Geometry: see drawing. Coordinates: mm, zero at the bounding-box minimum. Coordinates: 2 decimals unless noted, no trailing zeros. Write each loop counter-clockwise with the first axis right and the second up, starting at its lowest first coordinate (ties: lowest second). Pieces come first, ordered by that corner, then holes. Notation, with made-up numbers: (12, 86.25) - (62, 86.25) arc R9 cw to (62, 101.25) - close; hole circle Ø4 at (-12, 83). An arc over 180 degrees is marked (long way). Use CSV: the item, a comma, the result in double quotes.
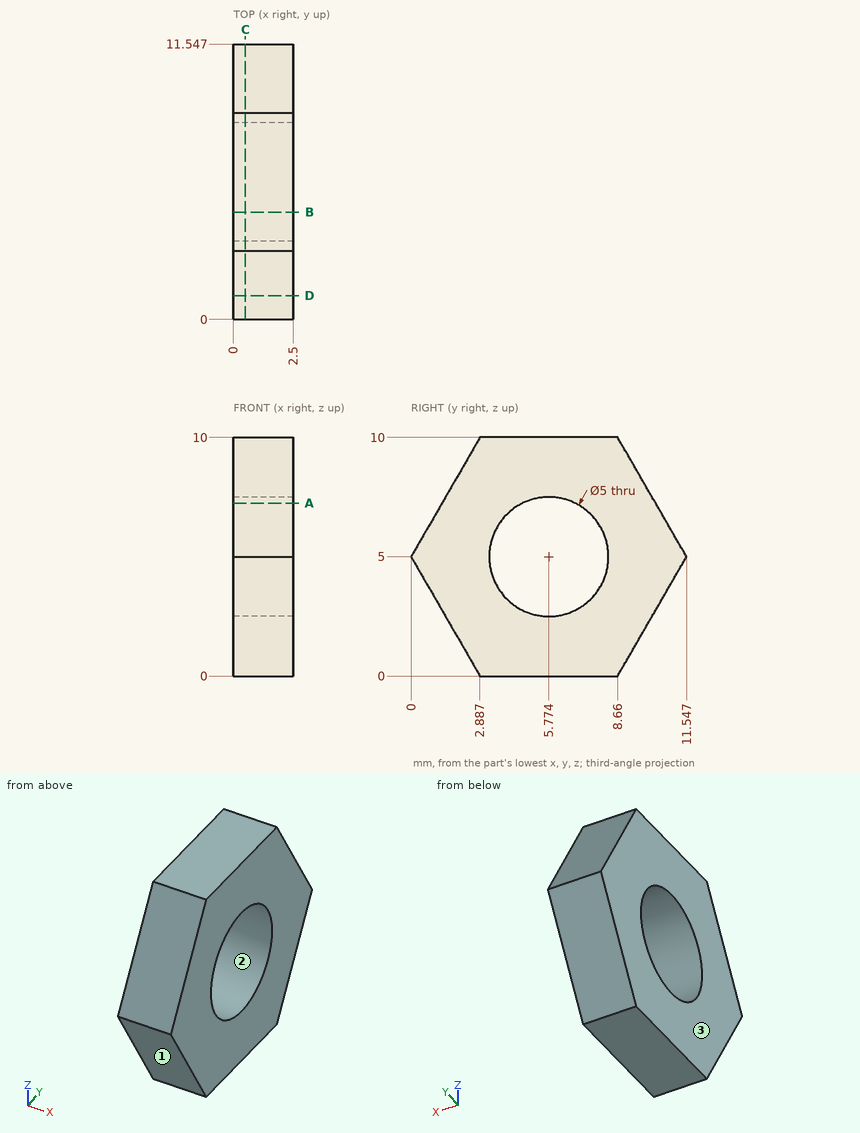
(1) Cut plane C-C on x = 0.5. Return loops of the section in (y, z).
Check values:
outline,"(0, 5) - (2.89, 0) - (8.66, 0) - (11.55, 5) - (8.66, 10) - (2.89, 10) - close; hole circle Ø5 at (5.77, 5)"
(2) Cut plane A-A on z = 7.25. Return loops of the section in (x, y).
Check values:
outline,"(0, 1.3) - (2.5, 1.3) - (2.5, 4.68) - (0, 4.68) - close; (0, 6.86) - (2.5, 6.86) - (2.5, 10.25) - (0, 10.25) - close"
(3) Cut plane D-D on y = 1. Return loops of the section in (x, z).
Check values:
outline,"(0, 3.27) - (2.5, 3.27) - (2.5, 6.73) - (0, 6.73) - close"
(4) Pin query (flat end, axial travel): pin 1 Ø4 at (y, z) = (3, 4.5) entering from -X; pin 2 Ø1 at (x, y) = (0.5, 10) entering from -Z (1 decimal); pin 3 Ø3 at (y, z) = (5.77, 5) entering from -X. Return the tip coordinate at first contact, or that it passes through.
Check values:
pin 1,"x = 0"
pin 2,"z = 1.5"
pin 3,"through"
(5) Ray query, probe 1 along Z at (x, y) = (1.1, 6.75); probe 2 along Z at (x, y) = (2.3, 7.75); probe 3 along Y at (x, z) = (2.05, 4.75) (1 decimal). Return the intervals inside material, ascending. Write a range as from..to.
Check values:
probe 1,"0..2.7, 7.3..10"
probe 2,"0..3.47, 6.53..10"
probe 3,"0.1..3.3, 8.3..11.4"
(6) Cut plane B-B on y = 4.5. Return loops of the section in (x, z).
Check values:
outline,"(0, 0) - (2.5, 0) - (2.5, 2.85) - (0, 2.85) - close; (0, 7.15) - (2.5, 7.15) - (2.5, 10) - (0, 10) - close"
(7) Draft query along Y for the marked faces 1, 2 and 3. Return one class per face: pulls with the +Y half, pulls with the -Y half, needs draft (parallel to the pull), parting line crosses it, or undercut.
Check values:
face 1,"pulls with the -Y half"
face 2,"undercut"
face 3,"needs draft"
